Source: CAD feature listing. Evaluate the final solid. Frame: model axes, mm. Round coordinates to 2 decimals unless told otherwise and drop trailing zeros. Write each loop counter-clockwise with the first axis right and the second up, starting at its lowest first coordinate (ties: lowest second). Pieces come first, ordered by that corner, then holes.
from build123d import *

# Parameters (mm, degrees)
SKETCH1_R           = 20
BOSS_EXTRUDE1_DEPTH = 25
SKETCH2_R           = 4
CUT_EXTRUDE1_DEPTH  = 25
FILLET1_R           = 2


with BuildPart() as part:
    # Sketch1 → Boss-Extrude1 (new body)
    with BuildSketch(Plane(origin=(0, 0, 0), x_dir=(1, 0, 0), z_dir=(0, 1, 0))):
        with Locations(Location((0, 0, 0), (0, 0, 270))):
            Circle(SKETCH1_R)
    extrude(amount=BOSS_EXTRUDE1_DEPTH)

    # Sketch2 → Cut-Extrude1 (cut)
    with BuildSketch(Plane(origin=(0, 25, 0), x_dir=(1, 0, 0), z_dir=(0, 1, 0))):
        with Locations((0, 20)):
            Circle(SKETCH2_R)
        with Locations((14.142135624, 14.142135624)):
            Circle(SKETCH2_R)
        with Locations((20, 0)):
            Circle(SKETCH2_R)
        with Locations((14.142135624, -14.142135624)):
            Circle(SKETCH2_R)
        with Locations((0, -20)):
            Circle(SKETCH2_R)
        with Locations((-14.142135624, -14.142135624)):
            Circle(SKETCH2_R)
        with Locations((-20, 0)):
            Circle(SKETCH2_R)
        with Locations((-14.142135624, 14.142135624)):
            Circle(SKETCH2_R)
    extrude(amount=-CUT_EXTRUDE1_DEPTH, mode=Mode.SUBTRACT)

    # Fillet1
    fillet1_edges = [part.edges().sort_by_distance(p)[0] for p in [
        (16.673542367, 12.5, -11.045043455),
        (11.045043455, 12.5, -16.673542367),
        (19.6, 12.5, 3.979949748),
        (19.6, 12.5, -3.979949748),
        (11.045043455, 12.5, 16.673542367),
        (16.673542367, 12.5, 11.045043455),
        (-3.979949748, 12.5, 19.6),
        (3.979949748, 12.5, 19.6),
        (-16.673542367, 12.5, 11.045043455),
        (-11.045043455, 12.5, 16.673542367),
        (-19.6, 12.5, -3.979949748),
        (-19.6, 12.5, 3.979949748),
        (-11.045043455, 12.5, -16.673542367),
        (-16.673542367, 12.5, -11.045043455),
        (3.979949748, 12.5, -19.6),
        (-3.979949748, 12.5, -19.6),
    ]]
    fillet(fillet1_edges, radius=FILLET1_R)


solid = part.part
1) Contact query for flat-ended pins moving along their axis: P1, Ø2, axis at x = -10, z = -10.5, coming from the -Y side; P2, Ø5, axis at x = -8, y = 15, coming from the -Z side; P3, Ø4, axis at y = 17, z = 9.5, coming from the +X side; P4, Ø5, axis at x = -0.5, y = 4.5, coming from the +Z side. Output: stop coordinate, or through.
Taken from the geometry:
P1: stops at y = 0
P2: stops at z = -19.19
P3: stops at x = 18.54
P4: stops at z = 17.35
2) Section query B-B on x = 12. Return the cut outline in (y, z).
Taken from the geometry:
outline: (0, -10.76) - (25, -10.76) - (25, 10.76) - (0, 10.76) - close
3) Material intervals for line 1 (X direction, y = 16.5, z = 17.5); line 2 (X direction, y = 5.25, z = 14); line 3 (Z direction, x = 0, y = 4.5), sorted ascending.
Taken from the geometry:
line 1: x = -9.63 to -3.12, 3.12 to 9.63
line 2: x = -10.14 to 10.14
line 3: z = -16 to 16
4) Pull-direction query (Z, two-part tool) for faces 1 (the face through (0, 25, 0)), 2 (the face through (11.36, 12.68, 11.27)), 3 (the face through (-7.678, 12.325, 18.468)); classes: released by +Z, released by -Z, zero draft, split by the parting line, or undercut.
Taken from the geometry:
face 1: zero draft
face 2: undercut
face 3: released by +Z
5) Section query A-A on z = -11.5. Return the cut outline in (x, y), then the cut area to 3 significant figures.
Taken from the geometry:
outline: (-11.14, 0) - (11.14, 0) - (11.14, 25) - (-11.14, 25) - close
area: 557 mm2
